from build123d import *

# Parameters (mm, degrees)
ESQUISSE1_W             = 20
ESQUISSE1_H             = 22
BOSS_EXTRU_1_DEPTH      = 12
ESQUISSE2_R             = 4
ENL_V_MAT_EXTRU_1_DEPTH = 26
ESQUISSE4_W             = 58.42
ESQUISSE4_H             = 22
ESQUISSE4_R             = 1.7
BOSS_EXTRU_2_DEPTH      = 3
ESQUISSE5_R             = 1.7
ENL_V_MAT_EXTRU_2_DEPTH = 3
ESQUISSE3_R             = 1.7
ENL_V_MAT_EXTRU_3_DEPTH = 27
ESQUISSE6_W             = 16
ESQUISSE6_H             = 5
ENL_V_MAT_EXTRU_4_DEPTH = 10


with BuildPart() as part:
    # Esquisse1 → Boss.-Extru.1 (new body)
    with BuildSketch(Plane.XY):
        with Locations((10, 11)):
            Rectangle(ESQUISSE1_W, ESQUISSE1_H)
    extrude(amount=BOSS_EXTRU_1_DEPTH)

    # Esquisse2 → Enlèv. mat.-Extru.1 (cut)
    with BuildSketch(Plane(origin=(0, 22, 0), x_dir=(1, 0, 0), z_dir=(0, 1, 0))):
        with Locations((10, -6)):
            Circle(ESQUISSE2_R)
    extrude(amount=-ENL_V_MAT_EXTRU_1_DEPTH, mode=Mode.SUBTRACT)

    # Esquisse4 → Boss.-Extru.2 (add)
    with BuildSketch(Plane.XY.offset(12)):
        with Locations((10, 11)):
            Rectangle(ESQUISSE4_W, ESQUISSE4_H)
        with Locations((-15.41, 18.2)):
            Circle(ESQUISSE4_R, mode=Mode.SUBTRACT)
        with Locations((35.41, 18.2)):
            Circle(ESQUISSE4_R, mode=Mode.SUBTRACT)
    extrude(amount=BOSS_EXTRU_2_DEPTH)

    # Esquisse5 → Enlèv. mat.-Extru.2 (cut)
    with BuildSketch(Plane.XY.offset(15)):
        with Locations((-11, 19.5)):
            Circle(ESQUISSE5_R)
        with Locations((-11, 2.2)):
            Circle(ESQUISSE5_R)
        with Locations((31, 2.2)):
            Circle(ESQUISSE5_R)
        with Locations((31, 19.5)):
            Circle(ESQUISSE5_R)
        with Locations((-8.5, 11)):
            Circle(ESQUISSE5_R)
        with Locations((28.5, 11)):
            Circle(ESQUISSE5_R)
    extrude(amount=-ENL_V_MAT_EXTRU_2_DEPTH, mode=Mode.SUBTRACT)

    # Esquisse3 → Enlèv. mat.-Extru.3 (cut)
    with BuildSketch(Plane(origin=(20, 0, 0), x_dir=(0, 0, -1), z_dir=(1, 0, 0))):
        with Locations((-6, 15)):
            Circle(ESQUISSE3_R)
        with Locations((-6, 7)):
            Circle(ESQUISSE3_R)
    extrude(amount=-ENL_V_MAT_EXTRU_3_DEPTH, mode=Mode.SUBTRACT)

    # Esquisse6 → Enlèv. mat.-Extru.4 (cut)
    with BuildSketch(Plane.XY.offset(15)):
        with Locations((10, 19.5)):
            Rectangle(ESQUISSE6_W, ESQUISSE6_H)
    extrude(amount=-ENL_V_MAT_EXTRU_4_DEPTH, mode=Mode.SUBTRACT)


solid = part.part
Could you check a few things on this model? Use its own coordinates, in mm. A direction names the side the tool comes from. Coordinates: 2 decimals unless noted, no trailing zeros. Write each loop counter-clockwise with the first axis right and the second up, starting at its lowest first coordinate (ties: lowest second). Pieces come first, ordered by that corner, then holes. Notation, with made-up numbers: (28, -11) - (44, -11) arc R31 ccw to (44, 20) - close; hole circle Ø10 at (82, -9.5). An arc over 180 degrees is marked (long way). Put each result on its own line as item: value. Start each with the question number.
Q1. Please list where these lines run through material, in increasing order: L1, parallel to Y at x = 5.25, z = 6; L2, parallel to Y at x = 35.41, z = 14.05; L3, parallel to X at y = 19, z = 13.25.
Q2. Thinking about a two-plate mould opening in Z: for faces 5 (the cylindrical face through (16.86, 5.34, 6.37)), 6 (the flat face through (10, 11, 15)), 7 (the cylindrical face through (16.86, 13.34, 6.37)), 8 (the cylindrical face through (32.62, 20.01, 13.52)), which applies, pulls with the +Z half, pulls with the -Z half, needs draft (parallel to the pull), parting line crosses it, or undercut?
Q3. I want a section at D-D on x = 31. Write out the boundary of the cut face in (y, z), plus the area to 3 significant figures.
Q4. Which directions (+Z, -Z, +X, -X, +Y, -Y) give clear straight access to the entire face, cutting with the end or side of a thin tool? Please do faces 1 (the flat face through (29, 9, 12)), 2 (the cylindrical face through (3.23, 6.35, 4.43)), 3 (the flat face through (4, 20, 5)), 4 (the flat face through (-10, 9, 12)).
Q5. I want a section at A-A on y = 15. Write out the boundary of the cut face in (x, z).
Q6. I want a section at B-B on x = 10. Write out the boundary of the cut face in (y, z), plus the area to 3 significant figures.
Q7. I want a section at C-C on y = 2.2. Write out the boundary of the cut face in (x, z).
Q8. I'm going to push flat-ended pins straight in: P1, Ø3.5, axis at y = 9.5, z = 7, coming from the +X side; P2, Ø2.5, axis at y = 19.5, z = 8.5, coming from the -X side; P3, Ø5.5, axis at x = -11, y = 2.2, coming from the -Z side; P4, Ø3, axis at x = 35.41, y = 18.2, coming from the -Z side. Where does each tip first touch, or does it pass through?
Checks:
1. L1: 0 to 5.3, 8.7 to 13.3, 16.7 to 17
1. L2: 0 to 16.5, 19.9 to 22
1. L3: -19.21 to -16.91, -13.91 to -12.62, -9.38 to 2, 18 to 29.38, 32.62 to 33.91, 36.91 to 39.21
2. face 5: undercut
2. face 6: pulls with the +Z half
2. face 7: undercut
2. face 8: needs draft
3. outline: (0, 12) - (0.5, 12) - (0.5, 15) - (0, 15) - close; (3.9, 12) - (17.8, 12) - (17.8, 15) - (3.9, 15) - close; (21.2, 12) - (22, 12) - (22, 15) - (21.2, 15) - close
3. area: 45.6 mm²
4. face 1: -Z, +X, +Y, -Y
4. face 2: +X, -X
4. face 3: +Z, +Y
4. face 4: -Z, -X, +Y, -Y
5. outline: (-19.21, 12) - (0, 12) - (0, 7.7) - (6.38, 7.7) arc R4 cw to (13.62, 7.7) - (20, 7.7) - (20, 12) - (39.21, 12) - (39.21, 15) - (-19.21, 15) - close; (0, 0) - (20, 0) - (20, 4.3) - (13.62, 4.3) arc R4 cw to (6.38, 4.3) - (0, 4.3) - close
6. outline: (0, 0) - (22, 0) - (22, 2) - (0, 2) - close; (0, 10) - (17, 10) - (17, 15) - (0, 15) - close
6. area: 129 mm²
7. outline: (-19.21, 12) - (-12.7, 12) - (-12.7, 15) - (-19.21, 15) - close; (-9.3, 12) - (0, 12) - (0, 0) - (20, 0) - (20, 12) - (29.3, 12) - (29.3, 15) - (-9.3, 15) - close; (32.7, 12) - (39.21, 12) - (39.21, 15) - (32.7, 15) - close; hole circle Ø8 at (10, 6)
8. P1: x = 20
8. P2: x = 0
8. P3: z = 12
8. P4: through
